```python
from build123d import *

# Parameters (mm, degrees)
SKETCH1_W           = 56
SKETCH1_H           = 85
SKETCH1_R           = 1.375
BOSS_EXTRUDE1_DEPTH = 1.6
FILLET1_R           = 3.5
SKETCH3_W           = 13.1
SKETCH3_H           = 19.189632287
SKETCH3_W_2         = 14.44866431
BOSS_EXTRUDE2_DEPTH = 16
SKETCH5_W           = 5
SKETCH5_H           = 51
BOSS_EXTRUDE3_DEPTH = 16


with BuildPart() as part:
    # Sketch1 → Boss-Extrude1 (new body)
    with BuildSketch(Plane(origin=(0, 0, 0), x_dir=(1, 0, 0), z_dir=(0, 1, 0))):
        with Locations((28, 42.5)):
            Rectangle(SKETCH1_W, SKETCH1_H)
        with Locations(Location((3.5, 3.5, 0), (0, 0, 270))):
            Circle(SKETCH1_R, mode=Mode.SUBTRACT)
        with Locations(Location((52.5, 3.5, 0), (0, 0, 270))):
            Circle(SKETCH1_R, mode=Mode.SUBTRACT)
        with Locations(Location((52.5, 61.5, 0), (0, 0, 270))):
            Circle(SKETCH1_R, mode=Mode.SUBTRACT)
        with Locations(Location((3.5, 61.5, 0), (0, 0, 270))):
            Circle(SKETCH1_R, mode=Mode.SUBTRACT)
    extrude(amount=BOSS_EXTRUDE1_DEPTH)

    # Fillet1
    fillet1_edges = [part.edges().sort_by_distance(p)[0] for p in [
        (0, 0.8, -85),
        (56, 0.8, -85),
        (56, 0.8, 0),
        (0, 0.8, 0),
    ]]
    fillet(fillet1_edges, radius=FILLET1_R)

    # Sketch3 → Boss-Extrude2 (add)
    with BuildSketch(Plane(origin=(0, 1.6, 0), x_dir=(1, 0, 0), z_dir=(0, 1, 0))):
        with Locations((8.438548035, 74.501533843)):
            Rectangle(SKETCH3_W, SKETCH3_H)
        with Locations((27, 74.501533843)):
            Rectangle(SKETCH3_W, SKETCH3_H)
        with Locations((45.75, 74.501533843)):
            Rectangle(SKETCH3_W_2, SKETCH3_H)
    extrude(amount=BOSS_EXTRUDE2_DEPTH)

    # Sketch5 → Boss-Extrude3 (add)
    with BuildSketch(Plane(origin=(0, 1.6, 0), x_dir=(1, 0, 0), z_dir=(0, 1, 0))):
        with Locations((3.5, 32.5)):
            Rectangle(SKETCH5_W, SKETCH5_H)
    extrude(amount=BOSS_EXTRUDE3_DEPTH)


solid = part.part
```
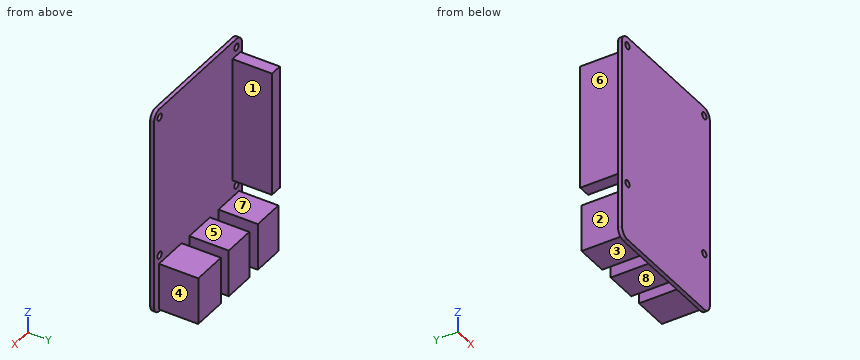
Source: CAD feature listing. Evaluate the final solid. Frame: model axes, mm. Face numbers are marked on the shaded views. A direction names the side the tool comes from. Coordinates: 2 decimals unless noted, no trailing zeros. Loops run counter-clockwise (first coordinate to the right, second up) from the corner with the lowest first, then second, coordinate; pieces in that order, holes last. Notation, with made-up numbers: M 2.5,-39.5 L 42.5,-39.5 A27 ccw 42.5,-10.5 Z; hole C 19,24 d2. An arc over 180 degrees is marked long. Put each result on its own line as item: value. Start each with the question number.
1) Pull-direction query (Z, two-part tool) for the marked faces 5, 6, 7 and 8; classes: pulls with the +Z half, pulls with the -Z half, needs draft (parallel to the pull), parting line crosses it, or undercut.
2) Ray query, L1, parallel to X at y = 13.75, z = -73.5; L2, parallel to X at y = 0.55, z = -61.5 (3 decimals); L3, parallel to Y at x = 22, z = -12. Return the intervals inside material, ascending. Write a range as from..to.
3) Cut plane B-B on z = -61.5. Return the cut outline in (x, y) (3 decimals), then the cut area to 3 significant figures.
4) Cut plane C-C on x = 25.5. Return the cut outline in (y, z), then the cut area to 3 significant figures.
5) Reachability of the marked faces 1, 2, 3 and 4 from +Z, -Z, +X, -X, +Y, -Y: full face, straight path, thin tool, end or side. Return the list, or none.
6) Cut plane D-D on z = -36. Return the cut outline in (x, y).
7) Cut plane A-A on y = 7. Return the cut outline in (x, z).
8) Contact query for flat-ended pins moving along their axis: pin 1 Ø5 at (y, z) = (6, -33) entering from +X; pin 2 Ø4.5 at (x, y) = (48, 11.5) entering from +Z; pin 3 Ø3.5 at (x, z) = (52.5, -3.5) entering from +Y. Output: stop coordinate, or through.
The answers:
1. face 5: pulls with the +Z half
1. face 6: needs draft
1. face 7: undercut
1. face 8: pulls with the -Z half
2. L1: x = 1.89..14.99, 20.45..33.55, 38.53..52.97
2. L2: x = 0..2.125, 4.875..51.125, 53.875..56
2. L3: y = 0..1.6
3. outline: M 0,0 L 2.125,0 L 2.125,1.6 L 0,1.6 Z; M 4.875,0 L 51.125,0 L 51.125,1.6 L 4.875,1.6 Z; M 53.875,0 L 56,0 L 56,1.6 L 53.875,1.6 Z
3. area: 80.8 mm²
4. outline: M 0,-85 L 1.6,-85 L 1.6,-84.1 L 17.6,-84.1 L 17.6,-64.91 L 1.6,-64.91 L 1.6,0 L 0,0 Z
4. area: 443 mm²
5. face 1: +Z, +X, +Y
5. face 2: -Z, -X, +Y
5. face 3: -Z, +X, -X, +Y
5. face 4: +Z, -Z, +X, +Y
6. outline: M 0,0 L 56,0 L 56,1.6 L 6,1.6 L 6,17.6 L 1,17.6 L 1,1.6 L 0,1.6 Z
7. outline: M 1,-58 L 6,-58 L 6,-7 L 1,-7 Z; M 1.89,-84.1 L 14.99,-84.1 L 14.99,-64.91 L 1.89,-64.91 Z; M 20.45,-84.1 L 33.55,-84.1 L 33.55,-64.91 L 20.45,-64.91 Z; M 38.53,-84.1 L 52.97,-84.1 L 52.97,-64.91 L 38.53,-64.91 Z
8. pin 1: stops at x = 6
8. pin 2: stops at z = -64.91
8. pin 3: stops at y = 1.6
